Geometry check sheet. Reference: drawing and pictorial views, mm from the part's lowest x, y, z. A direction names the side the tool comes from. Give positions to 0.01 mm unless a question says otherwise; leave off trailing zeros. Write each loop counter-clockwise with the first axis right and the second up, starting at its lowest first coordinate (ties: lowest second). Pieces come first, ordered by that corner, then holes. Notation, with made-up numbers: M -10.75,-20 L -1.75,-20 A7 ccw -1.75,-8 Z; hole C 82.5,73.5 d5. An arc over 180 degrees is marked long. Write item = value, one per line. Start each with the question number.
1) Access from +Z, -Z, +X, -X, +Y, -Y to the whole of each face (thin tool, end or side, straight path). Record for the marked faces 1 and 2.
2) Cross-section at D-D, the plane z = 4.75. Record the cut outline in (x, y).
3) Cross-section at C-C, the plane z = 0.5. Record the cut outline in (x, y).
4) Mould release check, pull along X, two halves, no side actions. Record for the marked faces 3, 4, 5 and 6: released by +X, released by -X, zero draft, split by the parting line, or undercut.
5) Scan lines: line 1 along Y through (x, z) = (11, 6.6); line 2 along Y through (x, z) = (11, 2.5); line 3 along X through (y, z) = (13.75, 6.25). Record each from-to range of solid material in increasing order. Write a range as [from, to].
6) Go/stop test with flat-tipped pins: pin 1 (4 mm diameter, centred on y = 14.5, z = 4, fed in from -X); pin 2 (4 mm diameter, centred on x = 14, y = 3.5, fed in from +Z); pin 3 (2 mm diameter, centred on y = 16.5, z = 5.5, fed in from -X); pin 4 (3 mm diameter, centred on y = 5, z = 4.5, fed in from +X). Record where each tip stops, or that it passes through.
7) Cross-section at A-A, the plane x = 11. Record the cut outline in (y, z), plus the area to 3 significant figures.
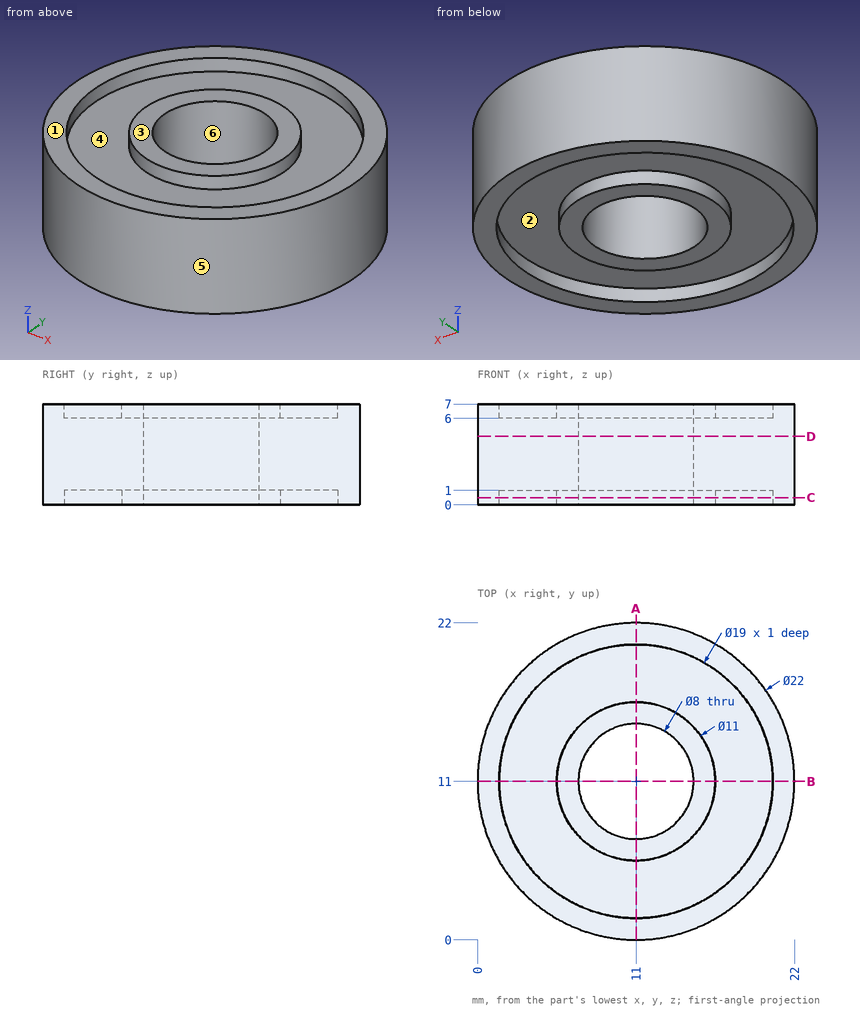
Reply:
q1.face_1 = +Z, +X, -X, +Y, -Y
q1.face_2 = -Z
q2.outline = C 11,11 d22; hole C 11,11 d8
q3.outline = C 11,11 d22; C 11,11 d11; hole C 11,11 d19; hole C 11,11 d8
q4.face_3 = zero draft
q4.face_4 = undercut
q4.face_5 = split by the parting line
q4.face_6 = undercut
q5.line_1 = [0, 1.5], [5.5, 7], [15, 16.5], [20.5, 22]
q5.line_2 = [0, 7], [15, 22]
q5.line_3 = [0.35, 1.91], [6.24, 8.1], [13.9, 15.76], [20.09, 21.65]
q6.pin_1 = 0.1
q6.pin_2 = 7
q6.pin_3 = 0.96
q6.pin_4 = 21.04
q7.outline = M 0,0 L 1.5,0 L 1.5,1 L 5.5,1 L 5.5,0 L 7,0 L 7,7 L 5.5,7 L 5.5,6 L 1.5,6 L 1.5,7 L 0,7 Z; M 15,0 L 16.5,0 L 16.5,1 L 20.5,1 L 20.5,0 L 22,0 L 22,7 L 20.5,7 L 20.5,6 L 16.5,6 L 16.5,7 L 15,7 Z
q7.area = 82.0 mm2
